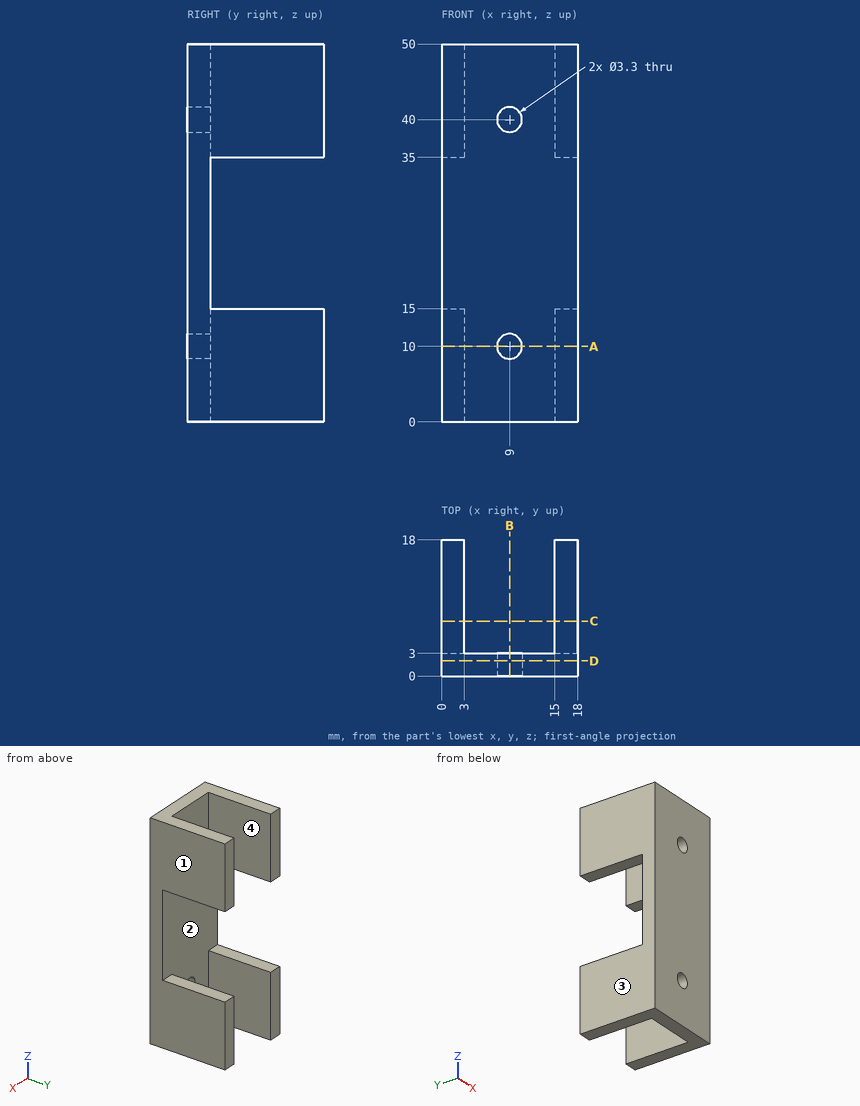
The figure shows three views and two pictorial views of one solid part (mm, origin at its lowest corner). Answer the questions. A direction names the side the tool comes from. Coordinates: 2 decimals unless noted, no trailing zeros. Loops run counter-clockwise (first coordinate to the right, second up) from the corner with the lowest first, then second, coordinate; pieces in that order, holes last.
(1) The part is cut by section C-C (y = 7.25). Determine the outline of the cut face in (x, z), and give its area (3 significant figures).
Solution:
outline: (0, 0) - (3, 0) - (3, 15) - (0, 15) - close; (0, 35) - (3, 35) - (3, 50) - (0, 50) - close; (15, 0) - (18, 0) - (18, 15) - (15, 15) - close; (15, 35) - (18, 35) - (18, 50) - (15, 50) - close
area: 180 mm2
(2) The part is cut by section A-A (z = 10). Determine the outline of the cut face in (x, y).
Solution:
outline: (0, 0) - (7.35, 0) - (7.35, 3) - (3, 3) - (3, 18) - (0, 18) - close; (10.65, 0) - (18, 0) - (18, 18) - (15, 18) - (15, 3) - (10.65, 3) - close
(3) The part is cut by section B-B (x = 9). Determine the outline of the cut face in (y, z), and give its area (3 significant figures).
Solution:
outline: (0, 0) - (3, 0) - (3, 8.35) - (0, 8.35) - close; (0, 11.65) - (3, 11.65) - (3, 38.35) - (0, 38.35) - close; (0, 41.65) - (3, 41.65) - (3, 50) - (0, 50) - close
area: 130 mm2
(4) Flat-ended cylindrical pins translate along their axes: pin 1 Ø3.5 at (x, y) = (16.5, 7) entering from -Z; pin 2 Ø9 at (x, z) = (8.5, 13.5) entering from +Y; pin 3 Ø1 at (x, y) = (4.5, 7.5) entering from +Z. Find the tip coordinate at first contact, or state that the pin passes through.
Solution:
pin 1: stops at z = 0
pin 2: stops at y = 3
pin 3: passes through
(5) Consider line 1 along X through (y, z) = (1.3, 40); line 2 along X through (y, z) = (3.5, 48.5); line 3 along Z through (x, y) = (1.5, 16.75). Determine where each line is inside the solid, lowest interval first.
Solution:
line 1: x = 0 to 7.35, 10.65 to 18
line 2: x = 0 to 3, 15 to 18
line 3: z = 0 to 15, 35 to 50
(6) The part is cut by section D-D (y = 2). Determine the outline of the cut face in (x, z), and give its area (3 significant figures).
Solution:
outline: (0, 0) - (18, 0) - (18, 50) - (0, 50) - close; hole circle Ø3.3 at (9, 10); hole circle Ø3.3 at (9, 40)
area: 883 mm2
(7) A tool of negligible diameter and unlimited length cuts with its end or side. For the marked faces 3 and 4, from which of +Z, -Z, +X, -X, +Y, -Y can it reach the whole face along a straight path? Write none if from no direction.
Solution:
face 3: +Z, -Z, -X, +Y, -Y
face 4: +Z, -Z, +Y
(8) The mould has two halves that part along Z. Classify the marked faces 1 and 2: released by +Z, released by -Z, zero draft, split by the parting line, or undercut.
Solution:
face 1: zero draft
face 2: undercut
